Work out the finished part from the listing and answer in its coordinate system (mm). A direction names the side the tool comes from. Give positions to 0.01 mm unless a question says otherwise; leave off trailing zeros. Loops run counter-clockwise (first coordinate to the right, second up) from the corner with the lowest first, then second, coordinate; pieces in that order, holes last. Notation, with made-up numbers: (-24, -8.75) - (10, -8.75) arc R13 cw to (10, -2.75) - close; hole circle Ø8 at (-24, 80). An arc over 180 degrees is marked (long way). One line per item, written item: value.
Autodesk Inventor part; units mm, degrees
ref_plane "Work Plane1" through (0, 0, -15) normal (0, 0, 1) x (1, 0, 0)
ref_plane "YZ Plane" through (0, 0, 0) normal (1, 0, 0) x (0, 1, 0)
ref_plane "XZ Plane" through (0, 0, 0) normal (0, 1, 0) x (-1, 0, 0)
sketch "Sketch1" plane through (0, 0, 0) normal (0, 0, 1) x (1, 0, 0)
  line L0 (0, 0) -> (25, 0)
  line L1 (25, 0) -> (25, 40)
  line L2 (25, 40) -> (0, 40)
  line L3 (0, 40) -> (0, 0)
  dimension "d1" = 25
  dimension "d2" = 40
  dimension "d3" = 25
extrude "Extrusion1" add sketch "Sketch1" against normal blind 30
sketch "Sketch2" plane through (25, 0, 0) normal (1, 0, 0) x (0, 0, -1)
  line L0 (0, 0) -> (30, 0)
  circle A0 centre (15, 6.56) radius 2.46
extrude "Extrusion2" cut sketch "Sketch2" against normal blind 30
sketch "Sketch3" plane through (0, 0, 0) normal (-1, 0, 0) x (0, 0, 1)
  line L0 (0, 0) -> (-30, 0)
  line L1 (-25.05, 0) -> (-4.95, 0)
  line L2 (-4.95, 0) -> (-4.95, 33.12)
  line L3 (-4.95, 33.12) -> (-25.05, 33.12)
  line L4 (-25.05, 33.12) -> (-25.05, 0)
  dimension "d11" = 20.1
extrude "Extrusion3" cut sketch "Sketch3" against normal blind 20
sketch "Sketch4" plane through (0, 0, 0) normal (0, -1, 0) x (1, 0, 0)
  line L0 (20, -4.95) -> (20, -25.05)
  line L1 (20, -15) -> (25, -15)
  line L2 (25, 0) -> (25, -30)
  line L3 (20, -8.025) -> (25, -8.025)
  line L4 (25, -8.025) -> (25, -21.975)
  line L5 (25, -21.975) -> (20, -21.975)
  line L6 (20, -21.975) -> (20, -8.025)
  line L7 (20, -8.025) -> (25, -21.975) construction
  line L8 (25, -8.025) -> (20, -21.975) construction
  line L9 (25, -12.54) -> (25, -17.46)
  point P0 (0, 0)
  point P1 (22.5, -15)
  dimension "d14" = 13.95
extrude "Extrusion4" add sketch "Sketch4" along normal blind 15
sketch "Sketch5" plane through (20, 0, 0) normal (-1, 0, 0) x (0, 0, 1)
  circle A0 centre (-15, 6.56) radius 2.46
  circle A1 centre (-15, 6.56) radius 4.7025
  circle A2 centre (-15, 6.56) radius 2.46
  circle A3 centre (-15, 6.56) radius 2.46
  point P0 (0, 0)
  dimension "d17" = 9.405
extrude "Extrusion5" cut sketch "Sketch5" against normal blind 2.1
sketch "Sketch6" plane through (25, 0, 0) normal (1, 0, 0) x (0, 0, -1)
  circle A0 centre (15, 6.56) radius 4.7025
  line L0 (15, 6.56) -> (15, 23.56)
  circle A1 centre (15, 23.56) radius 2.46
  point P0 (0, 0)
  dimension "d20" = 17
  dimension "d21" = 4.92
extrude "Extrusion6" cut sketch "Sketch6" against normal blind 10 contours A1
sketch "Sketch7" plane through (20, 0, 0) normal (-1, 0, 0) x (0, 0, 1)
  circle A0 centre (-15, 23.56) radius 2.46
  circle A1 centre (-15, 23.56) radius 4.7025
  point P0 (0, 0)
  dimension "d24" = 9.405
extrude "Extrusion7" cut sketch "Sketch7" against normal blind 2.1
sketch "Sketch9" plane through (25, 0, 0) normal (1, 0, 0) x (0, 0, -1)
  circle A0 centre (15, 6.56) radius 2.46
  circle A1 centre (15, 6.56) radius 2.46
  circle A2 centre (15, 23.56) radius 2.46
  circle A3 centre (15, 23.56) radius 2.46
  line L0 (30, 40) -> (30, 0)
  line L1 (30, 0) -> (30, 40)
  line L2 (30, 40) -> (0, 40)
  line L3 (0, 40) -> (0, 0)
  line L4 (0, 0) -> (8.025, 0)
  line L5 (21.975, 0) -> (21.975, -15)
  line L6 (21.975, -15) -> (8.025, -15)
  line L7 (8.025, -15) -> (8.025, 0)
  line L8 (0, 0) -> (8.025, 0)
  line L9 (21.975, 0) -> (30, 0)
extrude "Extrusion8" add sketch "Sketch9" along normal blind 5
sketch "Sketch10" plane through (0, 40, 0) normal (0, 1, 0) x (1, 0, 0)
  line L0 (0, 30) -> (30, 30)
  line L1 (30, 0) -> (0, 0)
  line L2 (0, 30) -> (30, 30)
  line L3 (30, 30) -> (30, 0)
  line L4 (30, 0) -> (0, 0)
  line L5 (0, 0) -> (0, 30)
extrude "Extrusion9" add sketch "Sketch10" along normal blind 30
sketch "Sketch12" plane through (30, 0, 0) normal (1, 0, 0) x (0, 0, -1)
  circle A0 centre (15, 6.56) radius 2.46
  line L0 (15, 6.56) -> (15, 15.06)
  circle A1 centre (15, 15.06) radius 2.525
  point P0 (0, 0)
  dimension "d31" = 8.5
  dimension "d33" = 5.05
extrude "Extrusion10" cut sketch "Sketch12" against normal blind 30 contours A1
sketch "Sketch14" plane through (0, 0, 0) normal (0, 0, 1) x (1, 0, 0)
  line L0 (30, 70) -> (0, 70)
  line L1 (0, 70) -> (0, 100)
  line L2 (30, 0) -> (30, 70)
  line L3 (30, 122.5) -> (30, 70)
  line L4 (30, 105) -> (30, 100)
  line L5 (-12, 145) -> (15, 145)
  line L6 (-7, 142.5) -> (-12, 145)
  line L7 (-7, 102.5) -> (-12, 100)
  line L8 (-7, 102.5) -> (-2, 122.5)
  line L9 (-2, 122.5) -> (-7, 142.5)
  line L10 (30, 122.5) -> (15, 145)
  line L11 (0, 100) -> (-12, 100)
  point P0 (0, 0)
  dimension "d86" = 12
extrude "Extrusion12" add sketch "Sketch14" against normal blind 30
sketch "Sketch15" plane through (0, 0, -25.05) normal (-1, 0, 0) x (0, 0, 1)
  line L0 (0, 33.12) -> (20.1, 33.12)
  line L1 (20.1, 33.12) -> (20.1, 0)
  line L2 (0, 33.12) -> (20.1, 33.12)
  line L3 (20.1, 33.12) -> (20.1, 31.1)
  line L4 (20.1, 31.1) -> (0, 31.1)
  line L5 (0, 31.1) -> (0, 33.12)
  point P0 (25.05, 0)
  dimension "d57" = 2.02
extrude "Extrusion13" add sketch "Sketch15" against normal blind 20
sketch "Sketch24" plane through (0, 0, 0) normal (0, 0, 1) x (1, 0, 0)
  line L0 (0, 100) -> (-12, 100)
  line L1 (-12, 100) -> (-7, 102.5)
  line L2 (0, 100) -> (-12, 100)
  line L3 (-12, 100) -> (-7, 102.5)
  line L4 (-7, 102.5) -> (-2, 122.5)
  line L5 (-7, 102.5) -> (-2, 122.5)
  line L6 (-2, 122.5) -> (-7, 142.5)
  line L7 (-2, 122.5) -> (-7, 142.5)
  line L8 (-7, 142.5) -> (-12, 145)
  line L9 (-7, 142.5) -> (-12, 145)
  line L10 (-12, 145) -> (15, 145)
  line L11 (-12, 145) -> (15, 145)
  line L12 (15, 145) -> (30, 122.5)
  line L13 (15, 145) -> (30, 122.5)
  line L14 (30, 122.5) -> (30, 87.5)
  line L15 (30, 87.5) -> (0, 87.5)
  line L16 (0, 87.5) -> (0, 100)
  point P0 (0, 0)
  dimension "d87" = 35
  dimension "d88" = 30
extrude "Extrusion14" add sketch "Sketch24" along normal blind 45
ref_plane "Work Plane1" through (0, 0, -15) normal (0, 0, 1) x (1, 0, 0)
mirror "Mirror1" about plane through (0, 0, -15) normal (0, 0, 1) of "Extrusion14"
properties part number "rec_b_40mm_x_120mm"
1. Section A-A (z = -15) is taken. Count the separate pieces of the cut face and the enclosed holes in it, and give its area (3 significant figures).
Output:
separate pieces: 4
enclosed holes: 0
area: 3,770 mm²
2. The mould has two halves that part along Z. Classify faces 5 (the cylindrical face through (21.035, 27.525, -12.472)), 6 (the flat face through (15, 0, -3)), 7 (the cylindrical face through (25.995, 7.502, -17.272)), 8 (the flat face through (25, -7, -21.975)): released by +Z, released by -Z, zero draft, split by the parting line, or undercut.
Output:
face 5: undercut
face 6: zero draft
face 7: undercut
face 8: released by -Z
3. Section D-D (z = 34) is taken. Write down the section's boundary in (x, y), and give its area (3 significant figures).
Output:
outline: (-12, 100) - (0, 100) - (0, 87.5) - (30, 87.5) - (30, 122.5) - (15, 145) - (-12, 145) - (-7, 142.5) - (-2, 122.5) - (-7, 102.5) - close
area: 1,780 mm²
4. For faces 1 (the flat face through (0, 62, -14)), 2 (the flat face through (-4.465, 112.64, -14.16)), 3 (the flat face through (22.1, 4.5, -13)), 4 (the flat face through (18, 0, -27)), determine the directions among +Z, -Z, +X, -X, +Y, -Y from which every point of the face is accessible in a straight line to the end or side of a thin tool.
Output:
face 1: +Z, -Z, -X, -Y
face 2: +Z, -Z, -X
face 3: -X
face 4: -Z, +X, -X, -Y
5. Section B-B (y = 15.06) is taken. Write down the section's boundary in (x, z) (3 decimals), and give its area (4 significant figures).
Output:
outline: (0, -30) - (30, -30) - (30, -17.525) - (20, -17.525) - (20, -25.05) - (0, -25.05) - close; (0, -4.95) - (20, -4.95) - (20, -12.475) - (30, -12.475) - (30, 0) - (0, 0) - close
area: 447.5 mm²
6. Find the intervals of material crossed by line 1 along Y through (x, z) = (27.25, -15) (3 decimals); line 2 along Y through (x, z) = (26, -15) (3 decimals); line 3 along Y through (x, z) = (10.5, -31.5), in increasing order.
Output:
line 1: y = -15 to 4.1, 9.02 to 12.535, 17.585 to 21.1, 26.02 to 126.625
line 2: y = -15 to 4.1, 9.02 to 12.535, 17.585 to 21.1, 26.02 to 128.5
line 3: y = 87.5 to 145
7. Section C-C (x = -4) is taken. Write down the section's boundary in (y, z).
Output:
outline: (100, -75) - (114.5, -75) - (114.5, 45) - (100, 45) - close; (130.5, -75) - (145, -75) - (145, 45) - (130.5, 45) - close
8. Flat-ended cylindrical pins translate along their axes: pin 1 Ø5 at (x, y) = (24.5, -5) entering from -Z (3 decimals); pin 2 Ø13 at (x, z) = (-3.5, -21) entering from -Y; pin 3 Ø8 at (y, z) = (23.56, -15) entering from -X. Find the tip coordinate at first contact, or state that the pin passes through.
Output:
pin 1: stops at z = -21.975
pin 2: stops at y = 0
pin 3: stops at x = 22.1
